For this review, take the finished solid that the model builds, in its own axes (mm). Give positions to 0.01 mm unless a question says otherwise; leave off trailing zeros. Write each loop counter-clockwise with the first axis right and the second up, starting at its lowest first coordinate (ties: lowest second). Pieces come first, ordered by that corner, then holes.
1) We need section D-D on y = -131.5. Give the boundary of the cut face in (x, z).
2) We need section A-A on x = -15. Give the boundary of the cut face in (y, z).
3) Wall thickness on line 1 along X through (y, z) = (405, 1.4); line 2 along X through (y, z) = (324.5, 0.65); line 3 along Y through (x, z) = (0.5, 1.6): over which ranges is each line inside the solid? List them lowest first.
4) We need section C-C on z = 1.7. Give the boundary of the cut face in (x, y).
5) For P1, Ø13, axis at x = -47.63, y = 377.5, coming from the -Z side; P2, Ø1, axis at x = -103.5, z = 1.5, coming from the -Y side; P3, Ø1, axis at y = -91, z = 1.5, coming from the +X side, all flat-tipped, find the tip position at first contact; note any pin that passes through.
6) We need section B-B on y = 350. Give the boundary of the cut face in (x, z).
7) Draft analysis for pull direction Y (two halves, no side actions). For faces 1 (the face through (-173.705, -182.904, 0.986)), 2 (the face through (-75, 236, 2)), 3 (the face through (-5.21, 310.34, 0.99)), state which applies: pulls with the +Y half, pulls with the -Y half, needs draft (parallel to the pull), parting line crosses it, or undercut.
Autodesk Inventor part; units mm, degrees
ref_plane "YZ Plane" through (0, 0, 0) normal (1, 0, 0) x (0, 1, 0)
ref_plane "XZ Plane" through (0, 0, 0) normal (0, 1, 0) x (-1, 0, 0)
ref_plane "XY Plane" through (0, 0, 0) normal (0, 0, 1) x (1, 0, 0)
sketch "Sketch1" plane through (0, 0, 0) normal (0, 0, 1) x (1, 0, 0)
  line L0 (-459.3004, -153.7378) -> (320, -153.7378)
  line L1 (320, -153.7378) -> (320, 670)
  line L2 (320, 670) -> (-459.3004, 670)
  line L3 (-459.3004, 670) -> (-459.3004, -153.7378)
  line L4 (120, -153.7378) -> (320, 0)
  circle A0 centre (0, 350) radius 40
  line L5 (320, 0) -> (120, 0)
  line L6 (120, 0) -> (120, -153.7378)
  line L7 (-459.3004, -153.7378) -> (-459.3004, -211.2657)
  line L8 (-459.3004, -211.2657) -> (120, -153.7378)
  point P0 (0, 0)
  dimension "d14" = 80
  dimension "d15" = 320
  dimension "d16" = 200
  dimension "d17" = 320
  dimension "d18" = 350
extrude "Plate1" add sketch "Sketch1" along normal blind 2 contours L3 L2 L1 L5 L6 L0 | L0 L8 L7
sketch "Sketch2" plane through (0, 0, 0) normal (0, 0, -1) x (-1, 0, 0)
  line L0 (-300, 650) -> (-100, 650) construction
  line L1 (-100, 650) -> (-100, 630) construction
  line L2 (-100, 630) -> (-300, 630) construction
  line L3 (-300, 630) -> (-300, 650) construction
  line L4 (-320, 670) -> (459.3004, 670)
  line L5 (-320, 0) -> (-320, 670)
  point P0 (0, 0)
  point P1 (-48, 100)
  point P2 (459.3004, 670)
  point P3 (-251, -525)
  point P4 (-50, 98)
  dimension "d6" = 200
  dimension "d9" = 20
  dimension "d10" = 20
  dimension "d11" = 20
mark "Mark1"
sketch "Sketch3" plane through (0, 0, 2) normal (0, 0, 1) x (1, 0, 0)
  circle A0 centre (0, 405) radius 5
  circle A1 centre (0, 350) radius 40
  point P0 (0, 0)
  dimension "d19" = 10
  dimension "d20" = 55
extrude "Cut1" cut sketch "Sketch3" against normal through all contours A0
pattern_circular "Circular Pattern1" count 6 over 360 about axis through (0, 350, 0) along (0, 0, 1) of "Cut1"
equation "\"d2\" = Thickness"
equation "\"BendReliefWidth\" = Thickness"
equation "\"BendReliefDepth\" = 0.5 * Thickness"
equation "\"CornerReliefSize\" = 4 * Thickness"
equation "\"MinimumRemnant\" = 2 * Thickness"
equation "\"TransitionRadius\" = BendRadius"
equation "\"JacobiRadiusSize\" = BendRadius"
equation "\"GapSize\" = Thickness"
properties part number "TRM 016 right board main+" material "AISI 304"
Results list:
1. outline: (-459.3, 0) - (120, 0) - (120, 2) - (-459.3, 2) - close
2. outline: (-167.14, 0) - (312.92, 0) - (312.92, 2) - (-167.14, 2) - close; (387.08, 0) - (670, 0) - (670, 2) - (387.08, 2) - close
3. line 1: x = -459.3 to -5, 5 to 320
3. line 2: x = -459.3 to -52.21, -43.05 to -30.82, 30.82 to 43.05, 52.21 to 320
3. line 3: y = -165.6 to 290.03, 299.97 to 310, 390 to 400.03, 409.97 to 670
4. outline: (-459.3, -211.27) - (120, -153.74) - (120, 0) - (320, 0) - (320, 670) - (-459.3, 670) - close; hole circle Ø10 at (-47.63, 322.5); hole circle Ø10 at (-47.63, 377.5); hole circle Ø80 at (0, 350); hole circle Ø10 at (0, 295); hole circle Ø10 at (0, 405); hole circle Ø10 at (47.63, 322.5); hole circle Ø10 at (47.63, 377.5)
5. P1: stops at z = 0
5. P2: stops at y = -175.98
5. P3: stops at x = 120
6. outline: (-459.3, 0) - (-40, 0) - (-40, 2) - (-459.3, 2) - close; (40, 0) - (320, 0) - (320, 2) - (40, 2) - close
7. face 1: pulls with the -Y half
7. face 2: needs draft
7. face 3: undercut
